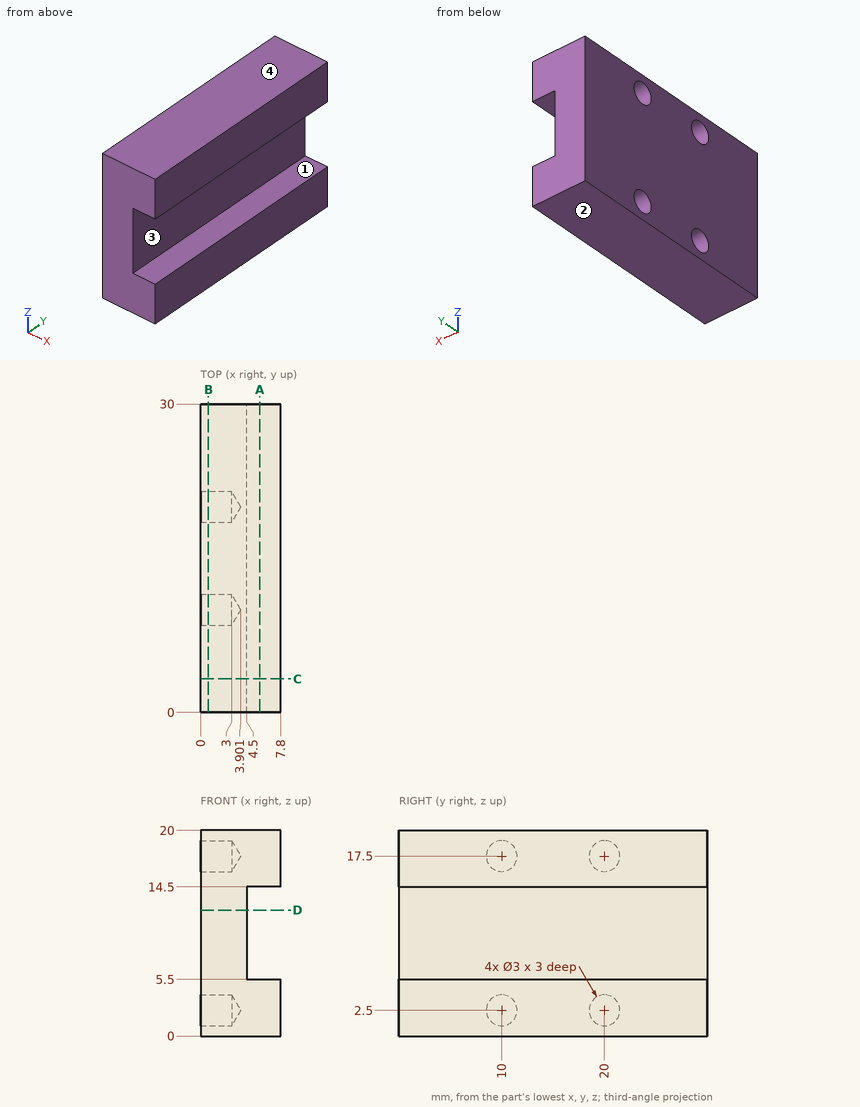
Geometry check sheet. Reference: drawing and pictorial views, mm from the part's lowest x, y, z. Round coordinates to 2 decimals unless told otherwise and drop trailing zeros. Loops run counter-clockwise (first coordinate to the right, second up) from the corner with the lowest first, then second, coordinate; pieces in that order, holes last. Notation, with made-up numbers: (70, 44) -> (86, 44) arc R16 ccw to (86, 55) -> close; hole circle Ø4 at (-10, 58). An arc over 180 degrees is marked (long way). Answer as a JSON object with one key per item and string values. Group by question number.
Item 1: Cross-section at D-D, the plane z = 12.25. Record the cut outline in (x, y).
Item 2: Cross-section at A-A, the plane x = 5.75. Record the cut outline in (y, z).
Item 3: Cross-section at C-C, the plane y = 3.25. Record the cut outline in (x, z), plus the area to 3 significant figures.
Item 4: Thickness scan on line 1 along Y through (x, z) = (2.2, 17.5); line 2 along Z through (x, y) = (1.6, 10); line 3 along Z through (x, y) = (5, 10.25). Record the ranges inside material, lowest first.
Item 5: Depth check by flat-ended pin: pin 1 Ø2.5 at (y, z) = (17, 8.5) entering from +X; pin 2 Ø1.8 at (y, z) = (20, 2.5) entering from -X. Enter the tip coordinate at first touch or a pass-through.
Item 6: Release check for a two-part mould opening along Z. For the marked faces 1, 2, 3 and 4 record: pulls with the +Z half, pulls with the -Z half, needs draft (parallel to the pull), parting line crosses it, or undercut.
Item 7: Cross-section at B-B, the plane x = 0.75. Record the cut outline in (y, z), plus the area to 3 significant figures.
Determined:
{
 "1": {"outline": "(0, 0) -> (4.5, 0) -> (4.5, 30) -> (0, 30) -> close"},
 "2": {"outline": "(0, 0) -> (30, 0) -> (30, 5.5) -> (0, 5.5) -> close; (0, 14.5) -> (30, 14.5) -> (30, 20) -> (0, 20) -> close"},
 "3": {"outline": "(0, 0) -> (7.8, 0) -> (7.8, 5.5) -> (4.5, 5.5) -> (4.5, 14.5) -> (7.8, 14.5) -> (7.8, 20) -> (0, 20) -> close", "area": "126 mm²"},
 "4": {"line 1": "y = 0 to 8.5, 11.5 to 18.5, 21.5 to 30", "line 2": "z = 0 to 1, 4 to 16, 19 to 20", "line 3": "z = 0 to 5.5, 14.5 to 20"},
 "5": {"pin 1": "stops at x = 4.5", "pin 2": "stops at x = 3.36"},
 "6": {"face 1": "undercut", "face 2": "pulls with the -Z half", "face 3": "undercut", "face 4": "pulls with the +Z half"},
 "7": {"outline": "(0, 0) -> (30, 0) -> (30, 20) -> (0, 20) -> close; hole circle Ø3 at (10, 2.5); hole circle Ø3 at (10, 17.5); hole circle Ø3 at (20, 2.5); hole circle Ø3 at (20, 17.5)", "area": "572 mm²"}
}
